The figure shows three views and two pictorial views of one solid part (mm, origin at its lowest corner). Answer the questions. Give positions to 0.01 mm unless a question says otherwise; leave off trailing zeros. Write each loop counter-clockwise with the first axis right and the second up, starting at its lowest first coordinate (ties: lowest second). Pieces come first, ordered by that corner, then holes. Notation, with made-up numbers: (-2, 69.5) -> (21, 69.5) arc R17 cw to (21, 74.5) -> close; hole circle Ø7 at (-23, 77). An arc over 180 degrees is marked (long way). Write each question's results on one line, items separated by ' | '. Start each with the question number.
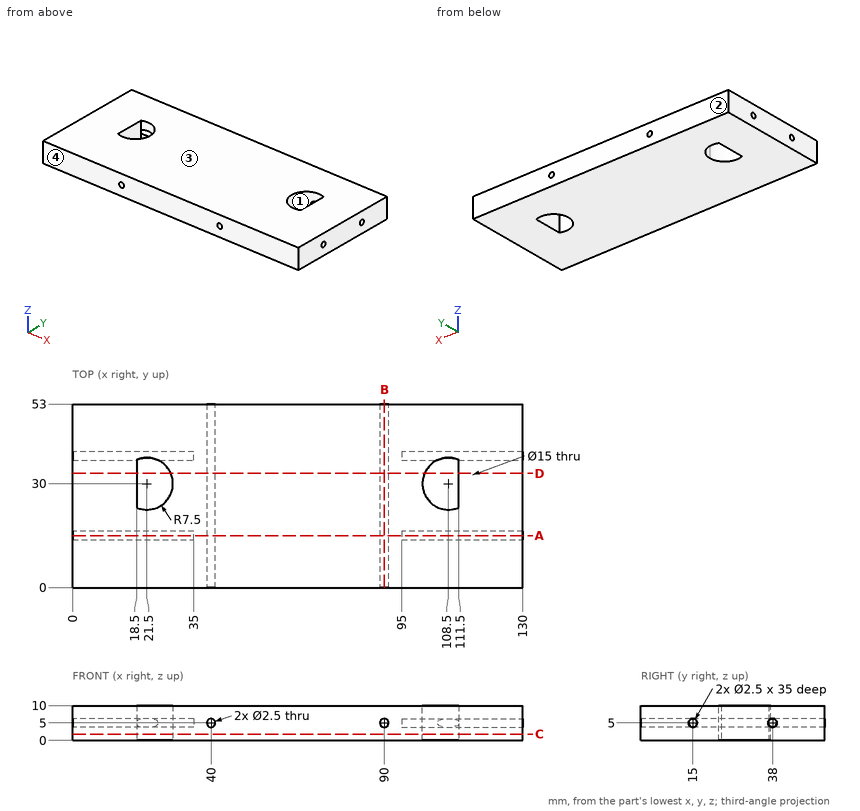
1. Each of these flat-tipped pins is pushed along its axis until it touches: pin 1 Ø0.8 at (y, z) = (15, 4.5) entering from -X; pin 2 Ø0.8 at (y, z) = (15, 5) entering from +X. Where does it stop, or does it pass through?
2. Section A-A (y = 15) is taken. Write down the section's boundary in (x, z).
3. Section B-B (x = 90) is taken. Write down the section's boundary in (y, z).
4. The mould has two halves that part along Y. Classify the marked faces 1, 2, 3 and 4: pulls with the +Y half, pulls with the -Y half, needs draft (parallel to the pull), parting line crosses it, or undercut.
5. Section C-C (z = 1.75) is taken. Write down the section's boundary in (x, y), then the cut area to 3 significant figures.
6. Section D-D (y = 33) is taken. Write down the section's boundary in (x, z).
7. Consider probe 1 along Z at (x, y) = (107, 38); probe 2 along Y at (x, z) = (20, 4.75); probe 3 along X at (y, z) = (24.5, 8.75). Determine where each line is inside the solid, lowest interval first. Write a range as [from, to].
Results:
1) pin 1: stops at x = 35 | pin 2: stops at x = 95
2) outline: (0, 0) -> (130, 0) -> (130, 3.75) -> (95, 3.75) -> (95, 6.25) -> (130, 6.25) -> (130, 10) -> (0, 10) -> (0, 6.25) -> (35, 6.25) -> (35, 3.75) -> (0, 3.75) -> close; hole circle Ø2.5 at (40, 5); hole circle Ø2.5 at (90, 5)
3) outline: (0, 0) -> (53, 0) -> (53, 3.75) -> (0, 3.75) -> close; (0, 6.25) -> (53, 6.25) -> (53, 10) -> (0, 10) -> close
4) face 1: undercut | face 2: pulls with the +Y half | face 3: needs draft | face 4: pulls with the -Y half
5) outline: (0, 0) -> (130, 0) -> (130, 53) -> (0, 53) -> close; hole (18.5, 23.13) arc R7.5 ccw to (29, 30) arc R7.5 ccw to (18.5, 36.87) -> close; hole (111.5, 23.13) -> (111.5, 36.87) arc R7.5 ccw (long way) to start | area: 6,630 mm²
6) outline: (0, 0) -> (18.5, 0) -> (18.5, 10) -> (0, 10) -> close; (28.37, 0) -> (101.63, 0) -> (101.63, 10) -> (28.37, 10) -> close; (111.5, 0) -> (130, 0) -> (130, 10) -> (111.5, 10) -> close; hole circle Ø2.5 at (40, 5); hole circle Ø2.5 at (90, 5)
7) probe 1: z = [0, 3.75], [6.25, 10] | probe 2: y = [0, 13.78], [16.22, 22.65], [39.22, 53] | probe 3: x = [0, 18.5], [26.6, 103.4], [111.5, 130]
